from build123d import *

# Parameters (mm, degrees)
EXTRUDE_1_DEPTH          = 2
SKETCH_2_W               = 56.4
SKETCH_2_H               = 71.9
EXTRUDE_3_DEPTH          = 15
SKETCH_6_R               = 3
CUT_EXTRUDE_1_DEPTH      = 18
SKETCH_7_W               = 10
SKETCH_7_H               = 8
SKETCH_7_H_2             = 11
EXTRUDE_4_DEPTH          = 3.7
SKETCH_8_R               = 1.5
CUT_EXTRUDE_2_DEPTH      = 6.7
CUT_EXTRUDE_5_DEPTH      = 1
CUT_EXTRUDE_5_DEPTH_BACK = 18
SKETCH_14_W              = 60.6
SKETCH_14_H              = 12.9
CUT_EXTRUDE_10_DEPTH     = 15
SKETCH_10_W              = 16.6
SKETCH_10_H              = 10
SKETCH_10_W_2            = 12.7
CUT_EXTRUDE_12_DEPTH     = 10
SKETCH_15_R              = 2.8
CUT_EXTRUDE_15_DEPTH     = 2.4


with BuildPart() as part:
    # 草图1 → 凸台-拉伸1 (new body)
    with BuildSketch(Plane.XY):
        with BuildLine():
            Line((0, 0), (8, 0))
            Line((8, 0), (8, 77))
            Line((8, 77), (0, 77))
            ThreePointArc((0, 77), (-5, 82), (0, 87))
            Line((0, 87), (79, 87))
            ThreePointArc((79, 87), (84, 82), (79, 77))
            Line((79, 77), (71, 77))
            Line((71, 77), (71, 0))
            Line((71, 0), (79, 0))
            ThreePointArc((79, 0), (84, -5), (79, -10))
            Line((79, -10), (71, -10))
            Line((71, -10), (62.339745962, -5))
            Line((62.339745962, -5), (16.660254038, -5))
            Line((16.660254038, -5), (8, -10))
            Line((8, -10), (0, -10))
            ThreePointArc((0, -10), (-5, -5), (0, 0))
        make_face()
    extrude(amount=EXTRUDE_1_DEPTH)

    # 草图2 → 凸台-拉伸3 (add)
    with BuildSketch(Plane.XY.offset(2)):
        with BuildLine():
            Line((8, 0), (0, 0))
            ThreePointArc((0, 0), (-5, -5), (0, -10))
            Line((0, -10), (8, -10))
            Line((8, -10), (16.660254038, -5))
            Line((16.660254038, -5), (62.339745962, -5))
            Line((62.339745962, -5), (71, -10))
            Line((71, -10), (79, -10))
            ThreePointArc((79, -10), (84, -5), (79, 0))
            Line((79, 0), (71, 0))
            Line((71, 0), (71, 77))
            Line((71, 77), (79, 77))
            ThreePointArc((79, 77), (84, 82), (79, 87))
            Line((79, 87), (0, 87))
            ThreePointArc((0, 87), (-5, 82), (0, 77))
            Line((0, 77), (8, 77))
            Line((8, 77), (8, 0))
        make_face()
        with Locations((39.5, 45.05)):
            Rectangle(SKETCH_2_W, SKETCH_2_H, mode=Mode.SUBTRACT)
    extrude(amount=EXTRUDE_3_DEPTH)

    # 草图6 → 切除-拉伸1 (cut, through all)
    with BuildSketch(Plane.XY.offset(17)):
        with Locations((0, 82)):
            Circle(SKETCH_6_R)
        with Locations((0, -5)):
            Circle(SKETCH_6_R)
        with Locations((79, -5)):
            Circle(SKETCH_6_R)
        with Locations((79, 82)):
            Circle(SKETCH_6_R)
    extrude(amount=-CUT_EXTRUDE_1_DEPTH, mode=Mode.SUBTRACT)

    # 草图7 → 凸台-拉伸4 (add)
    with BuildSketch(Plane.XY.offset(2)):
        with Locations((62.7, 65.8)):
            Rectangle(SKETCH_7_W, SKETCH_7_H)
        with Locations((16.3, 66)):
            Rectangle(SKETCH_7_W, SKETCH_7_H)
        with Locations((48.7, 14.6)):
            Rectangle(SKETCH_7_W, SKETCH_7_H_2)
        with Locations((20.5, 14.6)):
            Rectangle(SKETCH_7_W, SKETCH_7_H_2)
    extrude(amount=EXTRUDE_4_DEPTH)

    # 草图8 → 切除-拉伸2 (cut, through all)
    with BuildSketch(Plane.XY.offset(5.7)):
        with Locations((63.7, 65.2)):
            Circle(SKETCH_8_R)
        with Locations((15.5, 66.5)):
            Circle(SKETCH_8_R)
        with Locations((20.7, 14.4)):
            Circle(SKETCH_8_R)
        with Locations((48.7, 14.4)):
            Circle(SKETCH_8_R)
    extrude(amount=-CUT_EXTRUDE_2_DEPTH, mode=Mode.SUBTRACT)

    # 草图11 → 切除-拉伸5 (cut, two sides)
    with BuildSketch(Plane.XY.offset(17)) as cut_extrude_5_sk:
        Polygon((-211.639949222, 234.867393752), (4, 87), (11, 82.2), (68, 82.2), (75, 87), (290.639949222, 234.867393752), (290.639949222, 757.802777275), (-211.639949222, 757.802777275), align=None)
    extrude(amount=CUT_EXTRUDE_5_DEPTH, mode=Mode.SUBTRACT)
    extrude(cut_extrude_5_sk.sketch, amount=-CUT_EXTRUDE_5_DEPTH_BACK, mode=Mode.SUBTRACT)

    # 草图14 → 切除-拉伸10 (cut)
    with BuildSketch(Plane.XY.offset(17)):
        with Locations((39.5, 2.65)):
            Rectangle(SKETCH_14_W, SKETCH_14_H)
    extrude(amount=-CUT_EXTRUDE_10_DEPTH, mode=Mode.SUBTRACT)

    # 草图10 → 切除-拉伸12 (cut)
    with BuildSketch(Plane.XZ.offset(-81)):
        with Locations((22.8, 12)):
            Rectangle(SKETCH_10_W, SKETCH_10_H)
        with Locations((52.15, 12)):
            Rectangle(SKETCH_10_W_2, SKETCH_10_H)
    extrude(amount=-CUT_EXTRUDE_12_DEPTH, mode=Mode.SUBTRACT)

    # 草图15 → 切除-拉伸15 (cut)
    with BuildSketch(Plane(origin=(0, 0, 0), x_dir=(-1, 0, 0), z_dir=(0, 0, -1))):
        with Locations((-15.5, 66.5)):
            Circle(SKETCH_15_R)
        with Locations((-20.7, 14.4)):
            Circle(SKETCH_15_R)
        with Locations((-48.7, 14.4)):
            Circle(SKETCH_15_R)
        with Locations((-63.7, 65.2)):
            Circle(SKETCH_15_R)
    extrude(amount=-CUT_EXTRUDE_15_DEPTH, mode=Mode.SUBTRACT)


solid = part.part
The listing builds one solid part. Answer for the finished solid, in the listing's coordinates (mm). A direction names the side the tool comes from. Round coordinates to 2 decimals unless told otherwise and drop trailing zeros. Loops run counter-clockwise (first coordinate to the right, second up) from the corner with the lowest first, then second, coordinate; pieces in that order, holes last. Notation, with made-up numbers: M -35,67 L 23,67 A12 cw 23,89 Z; hole C -7.75,67 d7. An arc over 180 degrees is marked long. Return JSON: item names as keys, results as strings.
Q1. Find the intervals of material crossed by line 1 along X through (y, z) = (14.5, 1.5); line 2 along Y through (x, z) = (59.5, 3.5); line 3 along Y through (x, z) = (18, 4), in increasing order. Write a range as from..to.
Results list:
{"line 1": "x = 8..17.9, 23.5..45.9, 51.5..71", "line 2": "y = -5..-3.8, 61.8..69.8, 81..82.2", "line 3": "y = -5..-3.8, 9.1..20.1, 62..70, 81..82.2"}
Q2. Find section D-D, the plane x = 77.5. Determine the outline of the cut face in (y, z).
Results list:
{"outline": "M -10,0 L -7.6,0 L -7.6,17 L -10,17 Z; M -2.4,0 L 0,0 L 0,17 L -2.4,17 Z; M 77,0 L 79.4,0 L 79.4,17 L 77,17 Z; M 84.6,0 L 87,0 L 87,17 L 84.6,17 Z"}
Q3. Each of these flat-tipped pins is pushed along its axis until it touches: pin 1 Ø8 at (y, z) = (57, 11.5) entering from +X; pin 2 Ø2.5 at (x, z) = (10, 10) entering from -Y; pin 3 Ø1.5 at (y, z) = (24, 4) entering from -X; pin 4 Ø12 at (x, y) = (38.5, 54.5) entering from -Z. Where does it stop, or does it pass through?
Results list:
{"pin 1": "stops at x = 71", "pin 2": "stops at y = -9.57", "pin 3": "stops at x = 8", "pin 4": "stops at z = 0"}
Q4. The mould has two halves that part along Y. Classify faces 1 (the face through (69, 35, 17)), 2 (the face through (75, -10, 8)), 3 (the face through (47.5, 13.5, 4.1)): released by +Y, released by -Y, zero draft, split by the parting line, or undercut.
Results list:
{"face 1": "zero draft", "face 2": "released by -Y", "face 3": "undercut"}
Q5. Which of the six approach directions +Z, -Z, +X, -X, +Y, -Y give full straight-line access (tool end or side, diameter ignored) to faces 4 (the face through (71, 38, 8)), 5 (the face through (8, 39, 8)), 6 (the face through (20, 9.1, 4))?
Results list:
{"face 4": "+Z, -Z, +X", "face 5": "+Z, -Z, -X", "face 6": "+Z"}
Q6. Find section B-B, the plane z = 13. State how many separate pieces and enclosed holes the cut face has, plus the area to 3 significant figures.
Results list:
{"separate pieces": "2", "enclosed holes": "4", "area": "1,020 mm2"}
Q7. Find section A-A, the plane x = 48.7. Determine the outline of the cut face in (y, z).
Results list:
{"outline": "M -5,0 L 11.6,0 L 11.6,2.4 L 12.9,2.4 L 12.9,5.7 L 9.1,5.7 L 9.1,2 L -3.8,2 L -3.8,17 L -5,17 Z; M 15.9,2.4 L 17.2,2.4 L 17.2,0 L 82.2,0 L 82.2,7 L 81,7 L 81,2 L 20.1,2 L 20.1,5.7 L 15.9,5.7 Z"}
Q8. Find section C-C, the plane y = 42.5. Determine the outline of the cut face in (x, z), plus the area to 3 significant figures.
Results list:
{"outline": "M 8,0 L 71,0 L 71,17 L 67.7,17 L 67.7,2 L 11.3,2 L 11.3,17 L 8,17 Z", "area": "225 mm2"}
